The model under review builds one solid part; all positions refer to its coordinate system, in mm. Face numbers are marked on the shaded views. A direction names the side the tool comes from. Coordinates: 2 decimals unless noted, no trailing zeros. Write each loop counter-clockwise with the first axis right and the second up, starting at its lowest first coordinate (ties: lowest second). Pieces come first, ordered by that corner, then holes.
1) Add section C-C, the plane y = 10.16. Give the number of separate pieces and of enclosed holes in the cut face, then the cut area to 3 significant figures.
2) For line 1 (X direction, y = 1.6, z = -152.4); line 2 (Z direction, x = 165.1, y = 2.3); line 3 (Y direction, x = 114, z = -124.5), list the stretches that pass through material, from the lowest coordinate up.
3) Add section D-D, the plane x = 41.5. State the section outline as (y, z) points.
4) Add section B-B, the plane z = -12.7. State the section outline as (x, y) points (3 decimals).
5) Add section A-A, the plane x = 114.3. State the section outline as (y, z) points (3 decimals), then the cut area to 3 significant figures.
6) Mouldability with a two-part tool opening along X and no side actions: class the marked faces 3, 4 and 5 as released by +X, released by -X, zero draft, split by the parting line, or undercut.
7) Machinability: for the marked faces 1 and 2, which of the approach directions +Z, -Z, +X, -X, +Y, -Y give a long, thin tool a straight path to every point of the face, cutting with its end or side? Answer none if there is none.
8) For P1, Ø6, axis at x = 110, y = 7, coming from the +Z side; P2, Ø4, axis at x = 13, z = -11.5, coming from the +Y side; P3, Ø3, axis at x = 104.5, z = -81, coming from the -Y side; P4, Ø12, axis at y = 9.5, z = -91, coming from the +X side, all flat-tipped, find the tip position at first contact; note any pin that passes through.
Autodesk Inventor part; units mm, degrees
ref_plane "YZ Plane" through (0, 0, 0) normal (1, 0, 0) x (0, 1, 0)
ref_plane "XZ Plane" through (0, 0, 0) normal (0, 1, 0) x (-1, 0, 0)
ref_plane "XY Plane" through (0, 0, 0) normal (0, 0, 1) x (1, 0, 0)
sketch "Sketch1" plane through (0, 0, 0) normal (0, 1, 0) x (-1, 0, 0)
  line L0 (0, 0) -> (0, -165.1)
  line L1 (0, -165.1) -> (-177.8, -165.1)
  line L2 (-177.8, -165.1) -> (-177.8, 0)
  line L3 (-177.8, 0) -> (0, 0)
  line L4 (0, 0) -> (-25.4, 0)
  line L5 (-177.8, 0) -> (-152.4, 0)
  line L6 (0, -165.1) -> (-25.4, -165.1)
  line L7 (-177.8, -165.1) -> (-152.4, -165.1)
  line L8 (-152.4, 0) -> (-152.4, -25.4)
  line L9 (-152.4, -165.1) -> (-152.4, -139.7)
  line L10 (-25.4, 0) -> (-25.4, -25.4)
  line L11 (-25.4, -165.1) -> (-25.4, -139.7)
  line L12 (-38.1, -38.1) -> (-139.7, -38.1)
  line L13 (-25.4, -25.4) -> (-38.1, -38.1)
  line L14 (-25.4, -25.4) -> (-7.439488, -25.4) construction
  line L15 (-152.4, -25.4) -> (-139.7, -38.1)
  line L16 (-177.8, -82.55) -> (0, -82.55)
  line L17 (-152.4, -165.1) -> (-152.4, -139.7)
  line L18 (-25.4, -165.1) -> (-25.4, -139.7)
  line L19 (-38.1, -127) -> (-139.7, -127)
  line L20 (-25.4, -139.7) -> (-38.1, -127)
  line L21 (-152.4, -139.7) -> (-139.7, -127)
  dimension "d1" = 165.1
  dimension "d2" = 177.8
  dimension "d3" = 25.4
  dimension "d4" = 25.4
  dimension "d6" = 25.4
  dimension "d7" = 25.4
  dimension "d10" = 25.4
  dimension "d11" = 25.4
  dimension "d12" = 25.4
  dimension "d13" = 25.4
  dimension "d16" = 101.6
  dimension "d17" = 135
  dimension "d18" = 135
extrude "Extrusion1" add sketch "Sketch1" along normal blind 2.54 contours L0 L16 L2 L3 L8 L15 L12 L13 L10 | L0 L1 L11 L20 L19 L21 L9 L2 L16
sketch "Sketch2" plane through (0, 2.54, 0) normal (0, 1, 0) x (1, 0, 0)
  line L0 (25.4, 139.7) -> (25.4, 165.1)
  line L1 (25.4, 165.1) -> (0, 165.1)
  line L2 (0, 165.1) -> (0, 0)
  line L3 (0, 0) -> (25.4, 0)
  line L4 (25.4, 0) -> (25.4, 25.4)
  line L5 (25.4, 25.4) -> (38.1, 38.1)
  line L6 (38.1, 38.1) -> (139.7, 38.1)
  line L7 (139.7, 38.1) -> (152.4, 25.4)
  line L8 (152.4, 25.4) -> (152.4, 0)
  line L9 (152.4, 0) -> (177.8, 0)
  line L10 (177.8, 0) -> (177.8, 165.1)
  line L11 (177.8, 165.1) -> (152.4, 165.1)
  line L12 (152.4, 165.1) -> (152.4, 139.7)
  line L13 (152.4, 139.7) -> (139.7, 127)
  line L14 (139.7, 127) -> (38.1, 127)
  line L15 (38.1, 127) -> (25.4, 139.7)
  line L16 (2.54, 2.54) -> (2.54, 162.56)
  line L17 (2.54, 162.56) -> (22.86, 162.56)
  line L18 (22.86, 162.56) -> (22.86, 138.647898)
  line L19 (22.86, 138.647898) -> (37.047898, 124.46)
  line L20 (37.047898, 124.46) -> (140.752102, 124.46)
  line L21 (140.752102, 124.46) -> (154.94, 138.647898)
  line L22 (154.94, 138.647898) -> (154.94, 162.56)
  line L23 (154.94, 162.56) -> (175.26, 162.56)
  line L24 (175.26, 162.56) -> (175.26, 2.54)
  line L25 (175.26, 2.54) -> (154.94, 2.54)
  line L26 (154.94, 2.54) -> (154.94, 26.452102)
  line L27 (154.94, 26.452102) -> (140.752102, 40.64)
  line L28 (140.752102, 40.64) -> (37.047898, 40.64)
  line L29 (37.047898, 40.64) -> (22.86, 26.452102)
  line L30 (22.86, 26.452102) -> (22.86, 2.54)
  line L31 (22.86, 2.54) -> (2.54, 2.54)
  line L32 (22.86, 2.54) -> (22.86, 0)
  line L33 (154.94, 2.54) -> (154.94, 0)
  line L34 (154.94, 162.56) -> (154.94, 165.1)
  line L35 (22.86, 162.56) -> (22.86, 165.1)
  dimension "d21" = 2.54
extrude "Extrusion2" add sketch "Sketch2" along normal blind 17.78 contours L15 L14 L13 L12 L11 L34 L22 L21 L20 L19 L18 L35 L1 L0 | L32 L30 L29 L28 L27 L26 L33 L9 L8 L7 L6 L5 L4 L3
sketch "Sketch3" plane through (154.94, 2.54, 0) normal (1, 0, 0) x (0, 0, -1)
  line L0 (165.1, 0) -> (0, 0)
  line L1 (26.452102, 0) -> (26.452102, 17.78)
  line L2 (0, 17.78) -> (0, 0)
  line L3 (38.1, -2.54) -> (38.1, 17.78)
  line L4 (0, 0) -> (38.1, 17.78)
  line L5 (38.1, 17.78) -> (0, 17.78)
  line L6 (165.1, -2.54) -> (165.1, 17.78)
  line L7 (165.1, 0) -> (165.1, 17.78)
  line L8 (127, -2.54) -> (127, 17.78)
  line L9 (165.1, 17.78) -> (127, 17.78)
  line L10 (127, 17.78) -> (165.1, 0)
  point P0 (0, -2.54)
  dimension "d24" = 17.78
extrude "Extrusion3" cut sketch "Sketch3" against normal blind 132.08 contours L2 L5 L1 L4 | L1 L5 L4 | L10 L9 L6
sketch "Sketch4" plane through (0, 2.54, 0) normal (0, 1, 0) x (1, 0, 0)
  line L0 (0, 0) -> (0, 25.4)
  line L1 (0, 165.1) -> (0, 0)
  line L2 (0, 25.4) -> (25.4, 25.4)
  line L3 (0, 0) -> (25.4, 0)
  line L4 (25.4, 25.4) -> (0, 0)
  line L5 (0, 25.4) -> (25.4, 0)
  circle A0 centre (12.7, 12.7) radius 4.445
  dimension "d27" = 25.4
  dimension "d28" = 25.4
  dimension "d29" = 8.89
sketch "Sketch4 outline for Extrusion4" plane through (0, 2.54, 0) normal (0, 1, 0) x (1, 0, 0)
  circle A0 centre (12.7, 12.7) radius 4.445
extrude "Extrusion4" add sketch "Sketch4 outline for Extrusion4" along normal blind 2.54 draft -10
sketch "Sketch5" plane through (12.7, 5.08, -12.7) normal (0, 1, 0) x (1, 0, 0)
  circle A0 centre (0, 0) radius 3.997129
  line L0 (0, -3.997129) -> (0, 3.997129)
  line L1 (3.997129, 0) -> (-3.997129, 0)
  point P0 (-12.7, -12.7)
  dimension "d32" = 7.99426
  dimension "d33" = 7.99426
hole "Hole1" at (12.7, 5.08, -12.7) direction (0, -1, 0) diameter 4.9784 end through all
pattern_linear "Rectangular Pattern1" count 2 spacing 139.7 along (0, 0, -1) count 2 spacing 152.4 along (1, 0, 0) of "Hole1", "Extrusion4"
sketch "Sketch6" plane through (139.7, 0, -127) normal (0, 0, -1) x (-1, 0, 0)
  line L0 (101.6, 0) -> (101.6, 20.32)
  line L1 (0, 0) -> (0, 20.32)
  line L2 (101.6, 0) -> (0, 20.32)
  line L3 (0, 20.32) -> (0, 0)
  line L4 (0, 0) -> (101.6, 20.32)
  line L5 (50.8, 10.16) -> (76.2, 10.16)
  line L6 (50.8, 10.16) -> (25.4, 10.16)
  circle A0 centre (76.2, 10.16) radius 3.175
  circle A1 centre (25.4, 10.16) radius 3.175
  point P0 (139.7, 0)
  dimension "d48" = 101.6
  dimension "d49" = 22.6199
  dimension "d51" = 25.4
  dimension "d52" = 25.4
  dimension "d53" = 6.35
  dimension "d54" = 6.35
extrude "Extrusion5" cut sketch "Sketch6" against normal blind 88.9 contours A0 | A1
sketch "Sketch7" plane through (38.1, 0, -38.1) normal (0, 0, 1) x (1, 0, 0)
  circle A0 centre (25.4, 10.16) radius 3.175
  line L0 (25.4, 10.16) -> (22.225, 10.16)
  line L1 (22.225, 10.16) -> (22.225, 5.715)
  line L2 (22.225, 5.715) -> (25.4, 5.715)
  circle A1 centre (25.4, 5.715) radius 3.175
  line L3 (28.575, 5.715) -> (28.575, 15.875)
  line L4 (28.575, 15.875) -> (25.4, 15.875)
  circle A2 centre (25.4, 15.875) radius 3.175
  line L5 (22.225, 10.16) -> (22.225, 15.875)
  line L6 (25.4, 0) -> (25.4, 2.54)
  point P0 (-38.1, 0)
  point P1 (22.225, 13.0175)
  dimension "d58" = 6.35
  dimension "d57" = 4.445
  dimension "d60" = 6.35
  dimension "d61" = 6.35
  dimension "d62" = 5.715
  dimension "d63" = 2.54
  dimension "d64" = 3.175
  dimension "d65" = 13.335
extrude "Extrusion6" cut sketch "Sketch7" against normal blind 2.54
properties part number "ChairBaseBracket"
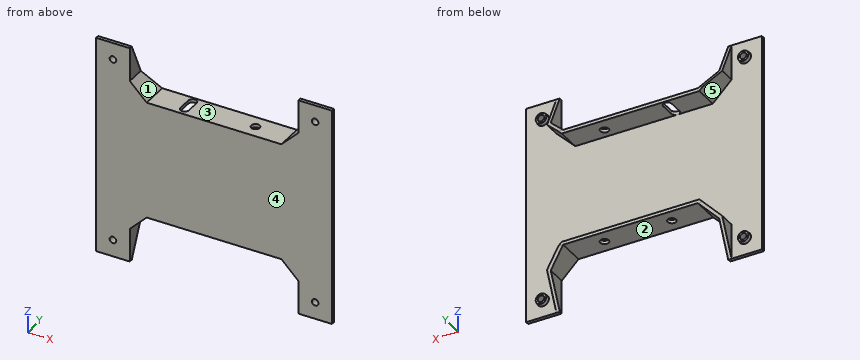
Geometry results:
1. separate pieces: 6
1. enclosed holes: 0
1. area: 748 mm2
2. line 1: x = 0 to 10.21, 15.19 to 25.4, 152.4 to 162.61, 167.59 to 177.8
2. line 2: z = -165.1 to -154.89, -149.91 to -15.19, -10.21 to 0
2. line 3: y = 0 to 7, 13.32 to 20.32
3. outline: (0, -127) - (20.32, -127) - (20.32, -124.46) - (2.54, -124.46) - (2.54, -40.64) - (20.32, -40.64) - (20.32, -38.1) - (0, -38.1) - close
4. outline: (0, 0) - (10.211, 0) - (10.211, 5.08) - (8.703, 5.08) - (8.255, 2.54) - (0, 2.54) - close; (15.189, 0) - (25.4, 0) - (25.4, 8.467) - (22.86, 8.467) - (22.86, 2.54) - (17.145, 2.54) - (16.697, 5.08) - (15.189, 5.08) - close; (152.4, 0) - (162.611, 0) - (162.611, 5.08) - (161.103, 5.08) - (160.655, 2.54) - (154.94, 2.54) - (154.94, 8.467) - (152.4, 8.467) - close; (167.589, 0) - (177.8, 0) - (177.8, 2.54) - (169.545, 2.54) - (169.097, 5.08) - (167.589, 5.08) - close
5. outline: (0, -127) - (6.985, -127) - (6.985, -124.46) - (2.54, -124.46) - (2.54, -40.64) - (6.985, -40.64) - (6.985, -38.1) - (0, -38.1) - close; (13.335, -127) - (20.32, -127) - (20.32, -124.46) - (13.335, -124.46) - close; (13.335, -40.64) - (20.32, -40.64) - (20.32, -38.1) - (13.335, -38.1) - close
5. area: 284 mm2
6. face 3: undercut
6. face 4: zero draft
6. face 5: released by -X
7. face 1: +Z, +Y, -Y
7. face 2: -Z, +Y, -Y
8. P1: stops at z = -38.1
8. P2: stops at y = 5.08
8. P3: stops at y = 0
8. P4: passes through
